CAD build for the part. Positions are in the model's coordinates, mm. Give positions to 0.01 mm unless a question says otherwise; leave off trailing zeros. Write each loop counter-clockwise with the first axis right and the second up, starting at its lowest first coordinate (ties: lowest second). Pieces come first, ordered by that corner, then holes. Notation, with made-up numbers: (-28, -25) - (-1, -25) arc R30 cw to (-1, 10) - close; hole circle Ø4 at (87.25, 11.25). An arc over 180 degrees is marked (long way). Answer as a JSON object with one key per item and string values.
from build123d import *

# Parameters (mm, degrees)
BOSS_EXTRUDE1_DEPTH         = 6.35
M3_CLEARANCE_HOLE1_D        = 3.4
TAP_DRILL_FOR_M3X0_5_TAP1_D = 2.5


with BuildPart() as part:
    # Sketch1 → Boss-Extrude1 (new body)
    with BuildSketch(Plane(origin=(0, 0, 0), x_dir=(1, 0, 0), z_dir=(0, 1, 0))):
        with BuildLine():
            Line((0, 0), (20, 0))
            ThreePointArc((20, 0), (27.5, 7.5), (20, 15))
            Line((20, 15), (0, 15))
            ThreePointArc((0, 15), (-7.5, 7.5), (0, 0))
        make_face()
    extrude(amount=BOSS_EXTRUDE1_DEPTH)

    # M3 Clearance Hole1 (through all)
    with Locations(Plane(origin=(0, 6.35, -7.5), x_dir=(0, 0, 1), z_dir=(0, 1, 0))):
        with Locations((0, 0), (0, 20)):
            Hole(M3_CLEARANCE_HOLE1_D / 2)

    # Tap Drill for M3x0.5 Tap1 (through all)
    with Locations(Plane(origin=(10, 6.35, -7.5), x_dir=(0, 0, 1), z_dir=(0, 1, 0))):
        with Locations((0, 0)):
            Hole(TAP_DRILL_FOR_M3X0_5_TAP1_D / 2)


solid = part.part
Item 1: Cut at C-C (z = -7.5). Give the cut face in (x, y), and give its area (3 significant figures).
Entries:
{"outline": "(-7.5, 0) - (-1.7, 0) - (-1.7, 6.35) - (-7.5, 6.35) - close; (1.7, 0) - (8.75, 0) - (8.75, 6.35) - (1.7, 6.35) - close; (11.25, 0) - (18.3, 0) - (18.3, 6.35) - (11.25, 6.35) - close; (21.7, 0) - (27.5, 0) - (27.5, 6.35) - (21.7, 6.35) - close", "area": "163 mm2"}
Item 2: Cut at A-A (x = 10). Give the cut face in (y, z), and give its area (3 significant figures).
Entries:
{"outline": "(0, -15) - (6.35, -15) - (6.35, -8.75) - (0, -8.75) - close; (0, -6.25) - (6.35, -6.25) - (6.35, 0) - (0, 0) - close", "area": "79.4 mm2"}
Item 3: Cut at D-D (x = -0.5). Give the cut face in (y, z), and give its area (3 significant figures).
Entries:
{"outline": "(0, -14.98) - (6.35, -14.98) - (6.35, -9.12) - (0, -9.12) - close; (0, -5.88) - (6.35, -5.88) - (6.35, -0.02) - (0, -0.02) - close", "area": "74.4 mm2"}
Item 4: Cut at B-B (y = 1). Give the cut face in (x, z), and give its area (3 significant figures).
Entries:
{"outline": "(0, -15) - (20, -15) arc R7.5 ccw to (20, 0) - (0, 0) arc R7.5 ccw to start; hole circle Ø3.4 at (0, -7.5); hole circle Ø2.5 at (10, -7.5); hole circle Ø3.4 at (20, -7.5)", "area": "454 mm2"}
Item 5: Mould opens along Z. For faces 1 (the flat face through (10, 0, -9)), 2 (the cylindrical face through (10.845, 3.131, -6.579)), 3 (the flat face through (10, 3, -15)), 4 (the cylindrical face through (-1.03, 3.13, -6.15)) say: +Z half, -Z half, draft (parallel to the pull), parting line (faces both ways), or undercut.
Entries:
{"face 1": "draft", "face 2": "undercut", "face 3": "-Z half", "face 4": "undercut"}
Item 6: Probe line 1 (X direction, y = 2.25, z = -7.5); line 2 (Z direction, x = -1, y = 3); line 3 (X direction, y = 3, z = -13). List the from-to ranges inside material, lowest first. Write a range as from..to.
Entries:
{"line 1": "-7.5..-1.7, 1.7..8.75, 11.25..18.3, 21.7..27.5", "line 2": "-14.93..-8.87, -6.13..-0.07", "line 3": "-5.1..25.1"}
